Check sheet for the drawn part. Datum: minimum x, y, z corner. Units: mm. Give positions to 0.01 mm unless a question says otherwise; leave off trailing zeros. Order: outer loops, then holes, each group sorted by start corner. A loop starts at its lowest first (then second) coordinate and runs counter-clockwise, first axis right, second up. Notation, with made-up numbers: M 42,82 L 66,82 A22 cw 66,116 Z; hole C 77.25,-7 d7. An arc over 180 degrees is marked long. Answer in a Markdown table with one row per item. Add a question column.
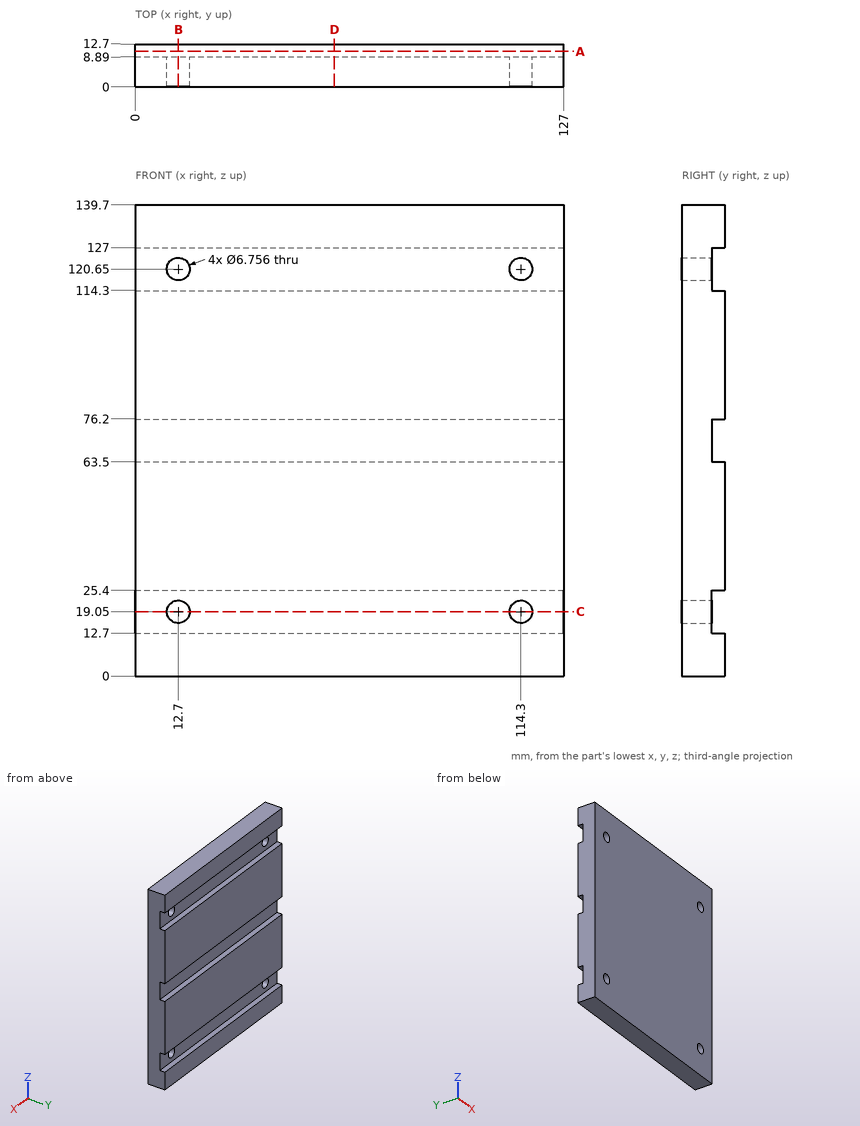
Q1. Go/stop test with a flat-tipped pin: pin 1 (6.5 mm diameter, centred on x = 45, z = 122.5, fed in from +Y). Record where the tip stops, or that it passes through.
Q2. Thickness scan on probe 1 along Z at (x, y) = (114.3, 3.75); probe 2 along Z at (x, y) = (105, 11); probe 3 along X at (y, z) = (4, 120.65). Record the ranges inside material, lowest first.
Q3. Cross-section at B-B (x = 12.7). Record the boundary of the cut face in (y, z), and give its area (3 significant figures).
Q4. Cross-section at A-A (y = 10.5). Record the boundary of the cut face in (x, z), and give its area (3 significant figures).
Q5. Cross-section at C-C (z = 19.05). Record the boundary of the cut face in (x, y).
Q6. Cross-section at D-D (x = 59). Record the boundary of the cut face in (y, z).
Values follow:
| question | item | result |
|---|---|---|
| 1 | pin 1 | y = 8.89 |
| 2 | probe 1 | 0 to 15.67, 22.43 to 117.27, 124.03 to 139.7 |
| 2 | probe 2 | 0 to 12.7, 25.4 to 63.5, 76.2 to 114.3, 127 to 139.7 |
| 2 | probe 3 | 0 to 9.32, 16.08 to 110.92, 117.68 to 127 |
| 3 | outline | M 0,0 L 12.7,0 L 12.7,12.7 L 8.89,12.7 L 8.89,15.67 L 0,15.67 Z; M 0,22.43 L 8.89,22.43 L 8.89,25.4 L 12.7,25.4 L 12.7,63.5 L 8.89,63.5 L 8.89,76.2 L 12.7,76.2 L 12.7,114.3 L 8.89,114.3 L 8.89,117.27 L 0,117.27 Z; M 0,124.03 L 8.89,124.03 L 8.89,127 L 12.7,127 L 12.7,139.7 L 0,139.7 Z |
| 3 | area | 1,510 mm² |
| 4 | outline | M 0,0 L 127,0 L 127,12.7 L 0,12.7 Z; M 0,25.4 L 127,25.4 L 127,63.5 L 0,63.5 Z; M 0,76.2 L 127,76.2 L 127,114.3 L 0,114.3 Z; M 0,127 L 127,127 L 127,139.7 L 0,139.7 Z |
| 4 | area | 12,900 mm² |
| 5 | outline | M 0,0 L 9.32,0 L 9.32,8.89 L 0,8.89 Z; M 16.08,0 L 110.92,0 L 110.92,8.89 L 16.08,8.89 Z; M 117.68,0 L 127,0 L 127,8.89 L 117.68,8.89 Z |
| 6 | outline | M 0,0 L 12.7,0 L 12.7,12.7 L 8.89,12.7 L 8.89,25.4 L 12.7,25.4 L 12.7,63.5 L 8.89,63.5 L 8.89,76.2 L 12.7,76.2 L 12.7,114.3 L 8.89,114.3 L 8.89,127 L 12.7,127 L 12.7,139.7 L 0,139.7 Z |
